Design review of the part shown in the three views and the two pictorial views. Dimensions are in mm from the part's minimum x, y and z. Round coordinates to 2 decimals unless told otherwise and drop trailing zeros. Order: outer loops, then holes, each group sorted by start corner. A loop starts at its lowest first (then second) coordinate and runs counter-clockwise, first axis right, second up.
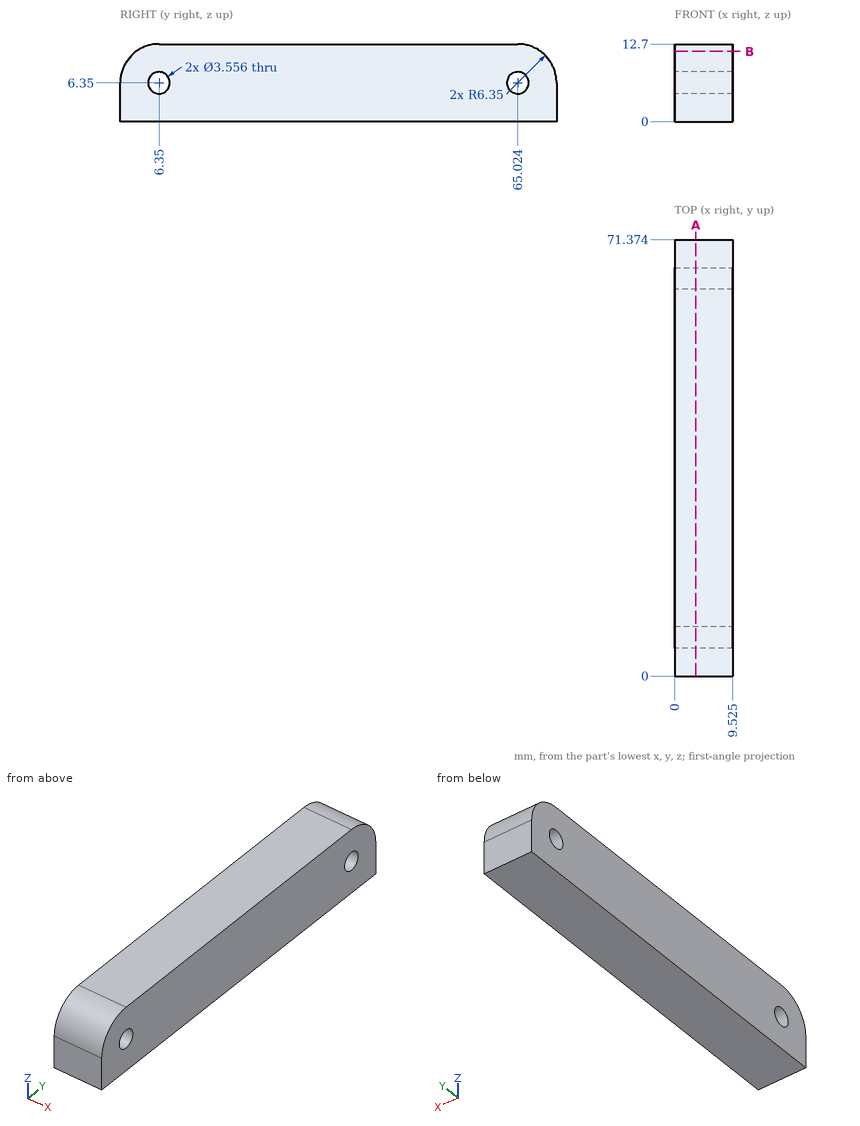
(1) Clearance check with a flat-ended pin moving along its axis: P1, Ø4, axis at x = 3, z = 9, coming from the +Y side. State where the tip first meets the part, or that it passes through.
(2) Add section B-B on z = 11.5. Give the boundary of the cut face in (x, y) (3 decimals).
(3) Wall thickness on L1, parallel to Y at x = 6.75, z = 6.75; L2, parallel to Z at x = 3, y = 6.35; L3, parallel to Y at x = 0.75, z = 5: over which ranges is each line inside the solid? List them lowest first.
(4) Add section A-A on x = 3.5. Give the boundary of the cut face in (y, z), plus the area to 3 significant figures.
Here are the results:
1. P1: stops at y = 71.34
2. outline: (0, 2.635) - (9.525, 2.635) - (9.525, 68.739) - (0, 68.739) - close
3. L1: y = 0.01 to 4.62, 8.08 to 63.29, 66.76 to 71.36
3. L2: z = 0 to 4.57, 8.13 to 12.7
3. L3: y = 0 to 5.19, 7.51 to 63.87, 66.18 to 71.37
4. outline: (0, 0) - (71.37, 0) - (71.37, 6.35) arc R6.35 ccw to (65.02, 12.7) - (6.35, 12.7) arc R6.35 ccw to (0, 6.35) - close; hole circle Ø3.56 at (6.35, 6.35); hole circle Ø3.56 at (65.02, 6.35)
4. area: 869 mm2
